Can you work these out from the model? Positions are in its coordinate system, mm. Face numbers are marked on the shaded views. A direction names the side the tool comes from. Give positions to 0.01 mm unless a question says otherwise; leave off trailing zeros. Loops run counter-clockwise (first coordinate to the right, second up) from the corner with the lowest first, then second, coordinate; pieces in that order, holes last. Notation, with made-up numbers: (54.5, 69.25) -> (95.5, 69.25) arc R10 ccw to (95.5, 78.25) -> close; hole circle Ø7 at (-16, 21). An arc over 180 degrees is marked (long way). Use CSV: the item, a comma, the result in double quotes.
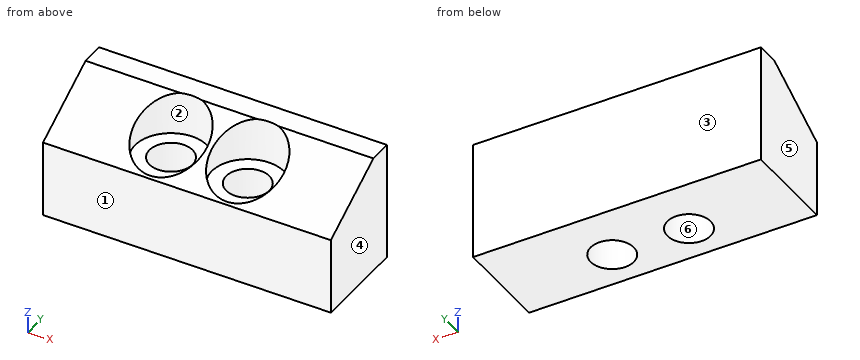
from build123d import *

# Parameters (mm, degrees)
F1_DEPTH       = 30
F3_D           = 9
F3_CBORE_D     = 15
F3_CBORE_DEPTH = 9


with BuildPart() as f1:
    # F0 (on Right) → F1 (new body, symmetric)
    with BuildSketch(Plane.YZ):
        Polygon((-20, 0), (0, 0), (0, 24.75), (-4.844555, 24.75), (-20, 16), align=None)
    extrude(amount=F1_DEPTH, both=True)

    # F3 (through all)
    with Locations(Plane.XY.offset(24.75)):
        with Locations((-8, -12), (8, -12)):
            CounterBoreHole(F3_D / 2, F3_CBORE_D / 2, F3_CBORE_DEPTH)


solid = f1.part
(1) Which directions (+Z, -Z, +X, -X, +Y, -Y) give clear straight access to the entire face, cutting with the end or side of a thin tool? Please do the marked faces 1 and 2.
Answer sheet:
face 1,"+Z, -Z, +X, -X, -Y"
face 2,"+Z"
(2) If we section it at D-D, the plane y = -5.75: Write out the boundary of the cut face in (x, z), then the cut area to 3 significant figures.
Answer sheet:
outline,"(-30, 0) -> (30, 0) -> (30, 24.23) -> (12.15, 24.23) -> (12.15, 15.75) -> (3.85, 15.75) -> (3.85, 24.23) -> (-3.85, 24.23) -> (-3.85, 15.75) -> (-12.15, 15.75) -> (-12.15, 24.23) -> (-30, 24.23) -> close"
area,"1,310 mm2"
(3) We'd pull the mould along X, two halves only. Please class the marked faces 3, 4, 5 and 6: released by +X, released by -X, zero draft, split by the parting line, or undercut.
Answer sheet:
face 3,"zero draft"
face 4,"released by +X"
face 5,"released by -X"
face 6,"undercut"
(4) If I drill on L1, parallel to X at y = -12, z = 19; L2, parallel to Y at x = 8, z = 7.25; L3, parallel to X at y = -11, z = 18.75, over which ranges is the centre line in solid material (lowest first)? Write a range as from..to.
Answer sheet:
L1,"x = -30..-15.5, -0.5..0.5, 15.5..30"
L2,"y = -20..-16.5, -7.5..0"
L3,"x = -30..-15.43, -0.57..0.57, 15.43..30"
(5) If we section it at B-B, the plane z = 2.75: Write out the boundary of the cut face in (x, y), then the cut area to 3 significant figures.
Answer sheet:
outline,"(-30, -20) -> (30, -20) -> (30, 0) -> (-30, 0) -> close; hole circle Ø9 at (-8, -12); hole circle Ø9 at (8, -12)"
area,"1,070 mm2"
(6) If we section it at A-A, the plane y = -8.5: Write out the boundary of the cut face in (x, z).
Answer sheet:
outline,"(-30, 0) -> (-10.83, 0) -> (-10.83, 15.75) -> (-14.63, 15.75) -> (-14.63, 22.64) -> (-30, 22.64) -> close; (-5.17, 0) -> (5.17, 0) -> (5.17, 15.75) -> (1.37, 15.75) -> (1.37, 22.64) -> (-1.37, 22.64) -> (-1.37, 15.75) -> (-5.17, 15.75) -> close; (10.83, 0) -> (30, 0) -> (30, 22.64) -> (14.63, 22.64) -> (14.63, 15.75) -> (10.83, 15.75) -> close"
(7) If we section it at C-C, the plane y = -12: Write out the boundary of the cut face in (x, z).
Answer sheet:
outline,"(-30, 0) -> (-12.5, 0) -> (-12.5, 15.75) -> (-15.5, 15.75) -> (-15.5, 20.62) -> (-30, 20.62) -> close; (-3.5, 0) -> (3.5, 0) -> (3.5, 15.75) -> (0.5, 15.75) -> (0.5, 20.62) -> (-0.5, 20.62) -> (-0.5, 15.75) -> (-3.5, 15.75) -> close; (12.5, 0) -> (30, 0) -> (30, 20.62) -> (15.5, 20.62) -> (15.5, 15.75) -> (12.5, 15.75) -> close"
(8) Will these pins go through, and if not, where does the flat tip stop? pin 1 Ø1 at (x, y) = (-20.5, -6.5) entering from +Z; pin 2 Ø1 at (x, y) = (-9, -8) entering from +Z; pin 3 Ø2 at (x, z) = (-19, 18.5) entering from -Y.
Answer sheet:
pin 1,"stops at z = 24.08"
pin 2,"stops at z = 15.75"
pin 3,"stops at y = -17.4"
